Design review of the part built by this model. Coordinates are the model's own, in mm. Coordinates: 2 decimals unless noted, no trailing zeros. Loops run counter-clockwise (first coordinate to the right, second up) from the corner with the lowest first, then second, coordinate; pieces in that order, holes last. Notation, with made-up numbers: (86, 3) -> (111, 3) arc R13 cw to (111, 18) -> close; hole circle Ø11 at (39, 43.25). An arc over 180 degrees is marked (long way). Answer in a Markdown table with one row per item.
```python
from build123d import *

# Parameters (mm, degrees)
ESBO_O1_W               = 10
ESBO_O1_H               = 213.5
FURO_COM_FOLGA_DE_M61_D = 6.6
ESBO_O7_R               = 80
CORTE_EXTRUS_O1_DEPTH   = 11
FURO_COM_FOLGA_DE_M62_D = 6.6


with BuildPart() as part:
    # Esboço1 → Revolução1 (revolve)
    with BuildSketch(Plane.XY):
        with Locations((0, 141.25)):
            Rectangle(ESBO_O1_W, ESBO_O1_H)
    revolve(axis=Axis((0, 0, 0), (1, 0, 0)))

    # Furo com folga de M61 (through all)
    with Locations(Plane.ZY.offset(18.8)):
        with Locations((0, 73.7), (73.7, 0), (0, -73.7), (-73.7, 0), (0, 0)):
            Hole(FURO_COM_FOLGA_DE_M61_D / 2)

    # Esboço7 → Corte-extrusão1 (cut, through all)
    with BuildSketch(Plane.ZY.offset(5)):
        with Locations((106.066017178, 106.066017178)):
            Circle(ESBO_O7_R)
        with Locations((106.066017178, -106.066017178)):
            Circle(ESBO_O7_R)
        with Locations((-106.066017178, -106.066017178)):
            Circle(ESBO_O7_R)
        with Locations((-106.066017178, 106.066017178)):
            Circle(ESBO_O7_R)
    extrude(amount=-CORTE_EXTRUS_O1_DEPTH, mode=Mode.SUBTRACT)

    # Furo com folga de M62 (through all)
    with Locations(Plane(origin=(14.343621622, 0, 0), x_dir=(0, 0, -1), z_dir=(1, 0, 0))):
        with Locations((0, 240.895271507), (240.895271507, 0), (0, -240.895271507), (-240.895271507, 0), (0, 0)):
            Hole(FURO_COM_FOLGA_DE_M62_D / 2)


solid = part.part
```
(1) To check wall thickness, follow probe 1 along Z at (x, y) = (-2.5, -116); probe 2 along Y at (x, z) = (0.75, 146.5); probe 3 along Z at (x, y) = (0.25, 81.5). State the ranges of each line that lie inside material, in increasing order.
Evaluation:
| item | result |
|---|---|
| probe 1 | z = -219.2 to -185.45, -26.69 to 26.69, 185.45 to 219.2 |
| probe 2 | y = -200.1 to -175.1, -37.04 to 37.04, 175.1 to 200.1 |
| probe 3 | z = -234.23 to -182.2, -29.93 to 29.93, 182.2 to 234.23 |
(2) Take a section at D-D on y = 15.5. Give the boundary of the cut face in (x, z).
Evaluation:
| item | result |
|---|---|
| outline | (-5, -247.52) -> (5, -247.52) -> (5, -30.82) -> (-5, -30.82) -> close; (-5, 30.82) -> (5, 30.82) -> (5, 247.52) -> (-5, 247.52) -> close |
(3) Take a section at B-B on z = -125. Give the boundary of the cut face in (x, y), and give its area (3 significant figures).
Evaluation:
| item | result |
|---|---|
| outline | (-5, -214.19) -> (5, -214.19) -> (5, -183.79) -> (-5, -183.79) -> close; (-5, -28.34) -> (5, -28.34) -> (5, 28.34) -> (-5, 28.34) -> close; (-5, 183.79) -> (5, 183.79) -> (5, 214.19) -> (-5, 214.19) -> close |
| area | 1,170 mm² |
(4) Take a section at A-A on y = -48. Give the boundary of the cut face in (x, z), and give its area (4 significant figures).
Evaluation:
| item | result |
|---|---|
| outline | (-5, -243.31) -> (5, -243.31) -> (5, -161.1) -> (-5, -161.1) -> close; (-5, -51.04) -> (5, -51.04) -> (5, 51.04) -> (-5, 51.04) -> close; (-5, 161.1) -> (5, 161.1) -> (5, 243.31) -> (-5, 243.31) -> close |
| area | 2,665 mm² |
(5) Take a section at C-C on x = -0.25. Count the separate pieces of the cut face and the enclosed holes in it, and give its area (3 significant figures).
Evaluation:
| item | result |
|---|---|
| separate pieces | 1 |
| enclosed holes | 13 |
| area | 109,000 mm² |
(6) For pin 1 (3 mm diameter, centred on x = -2, z = -32, fed in from +Y); pin 2 (4 mm diameter, centred on y = 240.9, z = 0, fed in from -X); pin 3 (5 mm diameter, centred on x = 4, z = 119, fed in from -Y); pin 4 (6 mm diameter, centred on x = 2.5, y = -170.5, fed in from +Z), all flat-tipped, find the tip position at first contact; note any pin that passes through.
Evaluation:
| item | result |
|---|---|
| pin 1 | stops at y = 246.12 |
| pin 2 | passes through |
| pin 3 | stops at y = -218.93 |
| pin 4 | stops at z = 182.89 |
(7) Draft analysis for pull direction Z (two halves, no side actions). For faces 1 (the cylindrical face through (0.07, -32.28, 245.89)), 2 (the cylindrical face through (-0.07, -136.706, -32.166)), 3 (the flat face through (5, -52, 3)), state which applies: pulls with the +Z half, pulls with the -Z half, needs draft (parallel to the pull), parting line crosses it, or undercut.
Evaluation:
| item | result |
|---|---|
| face 1 | parting line crosses it |
| face 2 | undercut |
| face 3 | needs draft |
